```python
from build123d import *

# Parameters (mm, degrees)
F0_R     = 6.35
F1_DEPTH = 50.8
F3_D     = 25.4


with BuildPart() as f1:
    # F0 (on Top) → F1 (new body)
    with BuildSketch(Plane.XY):
        Polygon((-50.8, 0), (0, 0), (0, 482.6034102367), (177.8, 660.4), (177.8, 711.2034102367), (0, 711.2034102367), (-50.8, 711.2034102367), (-228.6, 711.2034102367), (-228.6, 660.4034102367), (-50.8, 482.6034102367), align=None)
        with Locations((-203.2, 685.8034102367)):
            Circle(F0_R, mode=Mode.SUBTRACT)
        Polygon((-50.8, 533.4034102367), (-177.8, 660.4034102367), (-50.8, 660.4034102367), align=None, mode=Mode.SUBTRACT)
        Polygon((0, 660.4), (127, 660.4), (0, 533.4024358834), align=None, mode=Mode.SUBTRACT)
        with Locations((152.4, 685.8034102367)):
            Circle(F0_R, mode=Mode.SUBTRACT)
    extrude(amount=F1_DEPTH)

    # F3 (through all)
    with Locations(Plane(origin=(0, 0, 0), x_dir=(1, 0, 0), z_dir=(0, 0, -1))):
        with Locations((-25.4, -570.0667500496)):
            Hole(F3_D / 2)


solid = f1.part
```
Can you work these out from the model? Positions are in its coordinate system, mm. A direction names the side the tool comes from. Round coordinates to 2 decimals unless told otherwise and drop trailing zeros. Loops run counter-clockwise (first coordinate to the right, second up) from the corner with the lowest first, then second, coordinate; pieces in that order, holes last. Notation, with made-up numbers: M 55,-12.75 L 86,-12.75 A26 cw 86,8.25 Z; hole C -30.75,82 d1. An arc over 180 degrees is marked long. Answer as a JSON object with one key per item and string values. Group by question number.
Q1. Will these pins go through, and if not, where does the flat tip stop? pin 1 (12 mm diameter, centred on x = -80, z = 11.5, fed in from -Y); pin 2 (20.5 mm diameter, centred on x = -25.4, y = 570.07, fed in from -Z); pin 3 (3 mm diameter, centred on y = 146, z = 16.5, fed in from -X); pin 4 (15 mm diameter, centred on x = 85.5, z = 15.5, fed in from -Y).
Q2. Imagine slicing it at B-B, the plane z = 19.5. Please give me the cut outline in (x, y), then the cut area to 3 significant figures.
Q3. Please list where these lines run through material, in increasing order: L1, parallel to Y at x = -25.4, z = 16.5; L2, parallel to X at y = 534, z = 9; L3, parallel to X at y = 536, z = 24.
Q4. We'd pull the mould along Y, two halves only. Please class faces 6 (the flat face through (0, 596, 25)), 7 (the flat face through (-140.945, 572.748, 25.044)), 8 (the flat face through (-228.6, 686, 25)), 9 (the flat face through (-23, 711.203, 25)): +Y half, -Y half, draft (parallel to the pull), parting line (faces both ways), or undercut.
Q5. Imagine slicing it at D-D, the plane y = 147. Please give me the cut outline in (x, z).
Q6. Imagine slicing it at A-A, the plane x = -25.4. Please give me the cut outline in (y, z).
Q7. On a 3-axis mill with a long thin cutter (end or side, diameter ignored), from which of +Z, -Z, +X, -X, +Y, -Y can I reach the whole of each face in a straight line? I mean faces 1 (the flat face through (-115, 660.403, 25)), 2 (the flat face through (-26, 0, 25)), 3 (the flat face through (-41, 515, 0)), 4 (the flat face through (-50.8, 245, 25)), 5 (the flat face through (0, 238, 25)). Say none if no direction works.
Q8. Imagine slicing it at C-C, the plane x = -113.5. Please give me the cut outline in (y, z).
Findings:
{
 "1": {"pin 1": "stops at y = 505.8", "pin 2": "passes through", "pin 3": "stops at x = -50.8", "pin 4": "stops at y = 560.6"},
 "2": {"outline": "M -228.6,660.4 L -50.8,482.6 L -50.8,0 L 0,0 L 0,482.6 L 177.8,660.4 L 177.8,711.2 L -228.6,711.2 Z; hole C -203.2,685.8 d12.7; hole M -177.8,660.4 L -50.8,533.4 L -50.8,660.4 Z; hole C -25.4,570.07 d25.4; hole M 0,533.4 L 127,660.4 L 0,660.4 Z; hole C 152.4,685.8 d12.7", "area": "68,900 mm2"},
 "3": {"L1": "y = 0 to 557.37, 582.77 to 711.2", "L2": "x = -102.2 to -51.4, -50.8 to 0, 0.6 to 51.4", "L3": "x = -104.2 to -53.4, -50.8 to 0, 2.6 to 53.4"},
 "4": {"face 6": "undercut", "face 7": "-Y half", "face 8": "draft", "face 9": "+Y half"},
 "5": {"outline": "M -50.8,0 L 0,0 L 0,50.8 L -50.8,50.8 Z"},
 "6": {"outline": "M 0,0 L 557.37,0 L 557.37,50.8 L 0,50.8 Z; M 582.77,0 L 711.2,0 L 711.2,50.8 L 582.77,50.8 Z"},
 "7": {"face 1": "+Z, -Z", "face 2": "+Z, -Z, +X, -X, -Y", "face 3": "-Z, +X, -X, +Y, -Y", "face 4": "+Z, -Z, -X, -Y", "face 5": "+Z, -Z, +X, -Y"},
 "8": {"outline": "M 545.3,0 L 596.1,0 L 596.1,50.8 L 545.3,50.8 Z; M 660.4,0 L 711.2,0 L 711.2,50.8 L 660.4,50.8 Z"}
}
